from build123d import *

# Parameters (mm, degrees)
F1_DEPTH = 152.4
F2_R     = 34.925
F3_DEPTH = 101.6
F5_D     = 10.0838


with BuildPart() as f1:
    # F0 (on Front) → F1 (new body)
    with BuildSketch(Plane.XZ):
        with BuildLine():
            ThreePointArc((0, 6.35), (1.8598719395, 1.8598719395), (6.35, 0))
            Line((6.35, 0), (31.75, 0))
            ThreePointArc((31.75, 0), (36.2401280605, 1.8598719395), (38.1, 6.35))
            Line((38.1, 6.35), (38.1, 31.75))
            ThreePointArc((38.1, 31.75), (36.2401280605, 36.2401280605), (31.75, 38.1))
            Line((31.75, 38.1), (6.35, 38.1))
            ThreePointArc((6.35, 38.1), (1.8598719395, 36.2401280605), (0, 31.75))
            Line((0, 31.75), (0, 6.35))
        make_face()
        with BuildLine():
            Line((25.4, 6.35), (12.7, 6.35))
            ThreePointArc((12.7, 6.35), (8.2098719395, 8.2098719395), (6.35, 12.7))
            Line((6.35, 12.7), (6.35, 25.4))
            ThreePointArc((6.35, 25.4), (8.2098719395, 29.8901280605), (12.7, 31.75))
            Line((12.7, 31.75), (25.4, 31.75))
            ThreePointArc((25.4, 31.75), (29.8901280605, 29.8901280605), (31.75, 25.4))
            Line((31.75, 25.4), (31.75, 12.7))
            ThreePointArc((31.75, 12.7), (29.8901280605, 8.2098719395), (25.4, 6.35))
        make_face(mode=Mode.SUBTRACT)
    extrude(amount=F1_DEPTH)

    # F2 (on face) → F3 (join)
    with BuildSketch(Plane.XY.offset(38.1)):
        with Locations((19.05, -152.4)):
            Circle(F2_R)
    extrude(amount=-F3_DEPTH)

    # F5 (through all)
    with Locations(Plane.XY.offset(38.1)):
        with Locations((19.05, -38.1)):
            Hole(F5_D / 2)


solid = f1.part
Geometry check sheet. Reference: the model listing, model coordinates, mm. A direction names the side the tool comes from. Give positions to 0.01 mm unless a question says otherwise; leave off trailing zeros. Order: outer loops, then holes, each group sorted by start corner. A loop starts at its lowest first (then second) coordinate and runs counter-clockwise, first axis right, second up. Notation, with made-up numbers: (-9, -31) - (42, -31) arc R17 cw to (42, 0) - close; hole circle Ø5 at (-9, 26.25). An arc over 180 degrees is marked (long way). Use one line per item in the form item = value.
1) Access from +Z, -Z, +X, -X, +Y, -Y to the whole of each face (thin tool, end or side, straight path). Record for faces 5 (the face through (36.19, -60.7, 1.81)), 6 (the face through (19, -58, 6.35)), 7 (the face through (36.29, -60.7, 36.19)).
Working result:
face_5 = -Z, +X, +Y
face_6 = +Y
face_7 = +Z, +X, +Y
2) Depth check by flat-ended pin: pin 1 Ø12.5 at (x, y) = (24, -89.5) entering from -Z; pin 2 Ø4 at (y, z) = (-158.5, -7.5) entering from +X; pin 3 Ø2 at (x, z) = (13, 1) entering from -Y. Enter the tip coordinate at first touch or a pass-through.
Working result:
pin_1 = 0
pin_2 = 53.73
pin_3 = -186.96
3) Sectioned sample at C-C (y = -88). Record the boundary of the cut face in (x, z), and give its area (3 significant figures).
Working result:
outline = (0, 6.35) arc R6.35 ccw to (6.35, 0) - (31.75, 0) arc R6.35 ccw to (38.1, 6.35) - (38.1, 31.75) arc R6.35 ccw to (31.75, 38.1) - (6.35, 38.1) arc R6.35 ccw to (0, 31.75) - close; hole (6.35, 12.7) arc R6.35 ccw to (12.7, 6.35) - (25.4, 6.35) arc R6.35 ccw to (31.75, 12.7) - (31.75, 25.4) arc R6.35 ccw to (25.4, 31.75) - (12.7, 31.75) arc R6.35 ccw to (6.35, 25.4) - close
area = 806 mm^2
4) Draft check along Z on faces 1 (the face through (1.81, -60.7, 1.91)), 2 (the face through (19.232, -117.475, 19.228)), 3 (the face through (31.75, -59, 19)), 4 (the face through (1.91, -60.7, 36.29)). Enter one of: released by +Z, released by -Z, zero draft, split by the parting line, or undercut.
Working result:
face_1 = released by -Z
face_2 = undercut
face_3 = undercut
face_4 = released by +Z
5) Sectioned sample at A-A (y = -38.1). Record the boundary of the cut face in (x, z), and give its area (3 significant figures).
Working result:
outline = (0, 6.35) arc R6.35 ccw to (6.35, 0) - (14.01, 0) - (14.01, 6.35) - (12.7, 6.35) arc R6.35 cw to (6.35, 12.7) - (6.35, 25.4) arc R6.35 cw to (12.7, 31.75) - (14.01, 31.75) - (14.01, 38.1) - (6.35, 38.1) arc R6.35 ccw to (0, 31.75) - close; (24.09, 0) - (31.75, 0) arc R6.35 ccw to (38.1, 6.35) - (38.1, 31.75) arc R6.35 ccw to (31.75, 38.1) - (24.09, 38.1) - (24.09, 31.75) - (25.4, 31.75) arc R6.35 cw to (31.75, 25.4) - (31.75, 12.7) arc R6.35 cw to (25.4, 6.35) - (24.09, 6.35) - close
area = 678 mm^2
6) Sectioned sample at B-B (x = 19.05). Record the boundary of the cut face in (y, z) (3 decimals).
Working result:
outline = (-187.325, -63.5) - (-117.475, -63.5) - (-117.475, 0) - (-43.142, 0) - (-43.142, 6.35) - (-117.475, 6.35) - (-117.475, 31.75) - (-43.142, 31.75) - (-43.142, 38.1) - (-187.325, 38.1) - close; (-33.058, 0) - (0, 0) - (0, 6.35) - (-33.058, 6.35) - close; (-33.058, 31.75) - (0, 31.75) - (0, 38.1) - (-33.058, 38.1) - close
7) Material ranges on probe 1 along Y at (x, z) = (19.05, 3.75) (3 decimals); probe 2 along Z at (x, y) = (32, -21); probe 3 along X at (y, z) = (-38, 36), recorded low to high. Write a range as from..to.
Working result:
probe_1 = -187.325..-43.142, -33.058..0
probe_2 = 0..38.1
probe_3 = 1.63..14.01, 24.09..36.47
8) Sectioned sample at D-D (z = 2). Record the boundary of the cut face in (x, y) (3 decimals).
Working result:
outline = (1.724, -122.076) arc R34.925 ccw (long way) to (36.376, -122.076) - (36.376, 0) - (1.724, 0) - close; hole circle Ø10.084 at (19.05, -38.1)
